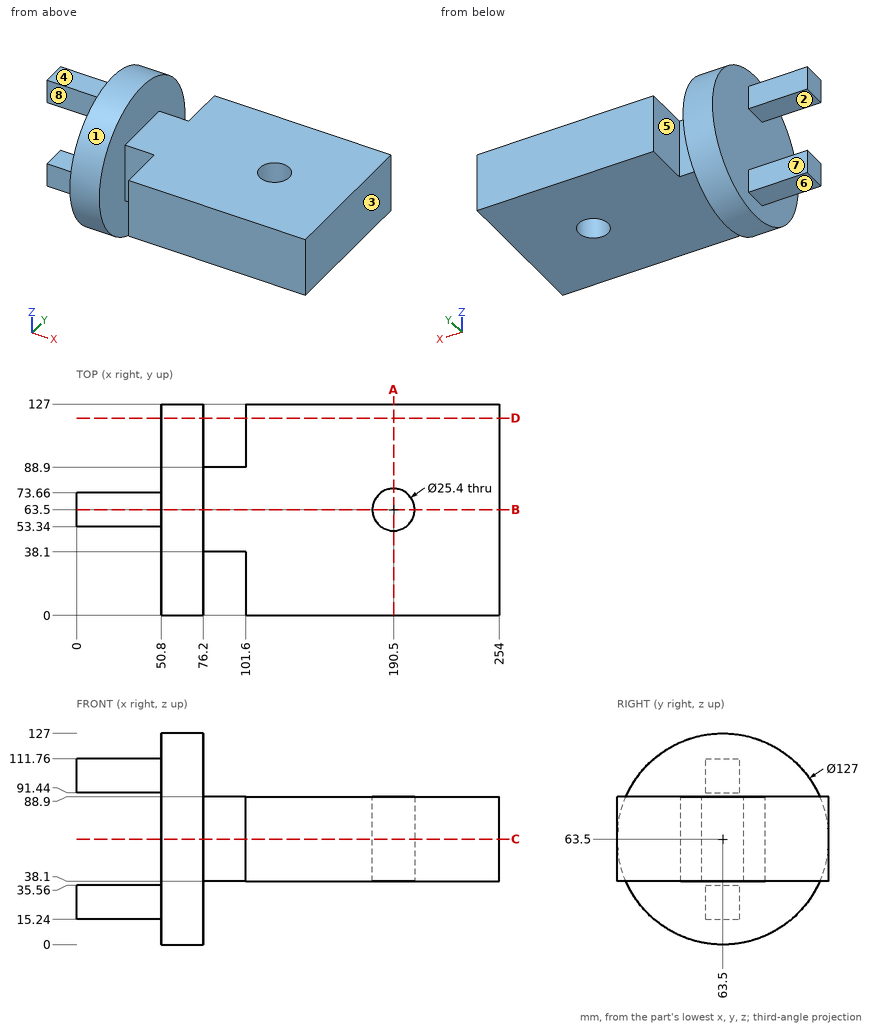
Geometry check sheet. Reference: drawing and pictorial views, mm from the part's lowest x, y, z. A direction names the side the tool comes from. Round coordinates to 2 decimals unless told otherwise and drop trailing zeros. Loops run counter-clockwise (first coordinate to the right, second up) from the corner with the lowest first, then second, coordinate; pieces in that order, holes last. Notation, with made-up numbers: (55.5, 44.25) - (86.5, 44.25) arc R22 cw to (86.5, 51.25) - close; hole circle Ø9 at (23.5, -22). An arc over 180 degrees is marked (long way). Use a Markdown table: item, result. Add a question column.
1. Section check B-B, the plane y = 63.5. Record the boundary of the cut face in (x, z), plus the area to 3 significant figures.
2. Section check C-C, the plane z = 63.5. Record the boundary of the cut face in (x, y), plus the area to 3 significant figures.
3. Section check D-D, the plane y = 118.5. Record the boundary of the cut face in (x, z).
4. Release check for a two-part mould opening along Z. For the marked faces 1, 2, 3 and 4 record: released by +Z, released by -Z, zero draft, split by the parting line, or undercut.
5. Section check A-A, the plane x = 190.5. Record the boundary of the cut face in (y, z).
6. Thickness scan on probe 1 along X at (y, z) = (63, 49); probe 2 along Y at (x, z) = (190, 64); probe 3 along X at (y, z) = (97.5, 17). Record the ranges inside material, lowest first. Write a range as [from, to].
7. Access from +Z, -Z, +X, -X, +Y, -Y to the whole of each face (thin tool, end or side, straight path). Record for the marked faces 5, 6, 7 and 8.
8. Gauge pin test, flat ends, axial feed: pin 1 (6 mm diameter, centred on x = 24.5, z = 27.5, fed in from +Y); pin 2 (10 mm diameter, centred on x = 15, y = 67.5, fed in from -Z); pin 3 (22.5 mm diameter, centred on x = 32.5, z = 28.5, fed in from -Y). Record the tip position at first contact, or that the pin passes through.
Checks:
| question | item | result |
|---|---|---|
| 1 | outline | (0, 15.24) - (50.8, 15.24) - (50.8, 0) - (76.2, 0) - (76.2, 38.1) - (177.8, 38.1) - (177.8, 88.9) - (76.2, 88.9) - (76.2, 127) - (50.8, 127) - (50.8, 111.76) - (0, 111.76) - (0, 91.44) - (50.8, 91.44) - (50.8, 35.56) - (0, 35.56) - close; (203.2, 38.1) - (254, 38.1) - (254, 88.9) - (203.2, 88.9) - close |
| 1 | area | 13,000 mm^2 |
| 2 | outline | (50.8, 0) - (76.2, 0) - (76.2, 38.1) - (101.6, 38.1) - (101.6, 0) - (254, 0) - (254, 127) - (101.6, 127) - (101.6, 88.9) - (76.2, 88.9) - (76.2, 127) - (50.8, 127) - close; hole circle Ø25.4 at (190.5, 63.5) |
| 2 | area | 23,400 mm^2 |
| 3 | outline | (50.8, 31.76) - (76.2, 31.76) - (76.2, 95.24) - (50.8, 95.24) - close; (101.6, 38.1) - (254, 38.1) - (254, 88.9) - (101.6, 88.9) - close |
| 4 | face 1 | split by the parting line |
| 4 | face 2 | undercut |
| 4 | face 3 | zero draft |
| 4 | face 4 | released by +Z |
| 5 | outline | (0, 38.1) - (50.8, 38.1) - (50.8, 88.9) - (0, 88.9) - close; (76.2, 38.1) - (127, 38.1) - (127, 88.9) - (76.2, 88.9) - close |
| 6 | probe 1 | x = [50.8, 177.81], [203.19, 254] |
| 6 | probe 2 | y = [0, 50.81], [76.19, 127] |
| 6 | probe 3 | x = [50.8, 76.2] |
| 7 | face 5 | +Z, -Z, +Y |
| 7 | face 6 | -Z, -X, +Y, -Y |
| 7 | face 7 | +Z, -Z, -X, +Y |
| 7 | face 8 | +Z, -Z, -X, -Y |
| 8 | pin 1 | stops at y = 73.66 |
| 8 | pin 2 | stops at z = 15.24 |
| 8 | pin 3 | stops at y = 53.34 |
